Design review of the part built by this model. Coordinates are the model's own, in mm. A direction names the side the tool comes from. Give positions to 0.01 mm unless a question says otherwise; leave off trailing zeros. Loops run counter-clockwise (first coordinate to the right, second up) from the corner with the lowest first, then second, coordinate; pieces in that order, holes last. Notation, with made-up numbers: (74, 68.5) - (80, 68.5) arc R22 cw to (80, 88.5) - close; hole circle Ø1 at (9.25, 70). An arc over 180 degrees is marked (long way). Write each question's results on one line, items separated by ' | '.
from build123d import *

# Parameters (mm, degrees)
F0_W      = 7.9375
F0_H      = 31.75
F0_R      = 2.38125
F1_DEPTH  = 9.525
F2_DEPTH  = 11.1125
F3_W      = 3.175
F3_H      = 2.38125
F4_DEPTH  = 3.175
F5_W      = 1.5875
F5_H      = 6.35
F6_DEPTH  = 6.35
F7_DEPTH  = 1.5875
F8_R      = 1.5875
F9_DEPTH  = 0.79375
F10_R     = 1.5875
F11_DEPTH = 0.79375


with BuildPart() as f1:
    # F0 (on Top) → F1 (new body)
    with BuildSketch(Plane.XY):
        Rectangle(F0_W, F0_H)
        with Locations((0, -11.90625)):
            Circle(F0_R, mode=Mode.SUBTRACT)
        with Locations((0, -3.96875)):
            Circle(F0_R, mode=Mode.SUBTRACT)
        with Locations((0, 3.96875)):
            Circle(F0_R, mode=Mode.SUBTRACT)
        with Locations((0, 11.90625)):
            Circle(F0_R, mode=Mode.SUBTRACT)
    extrude(amount=F1_DEPTH)

    # F0 (on Top) → F2 (join)
    with BuildSketch(Plane.XY):
        with Locations((0, 11.90625)):
            Circle(F0_R)
        with Locations((0, -11.90625)):
            Circle(F0_R)
        with Locations((0, 3.96875)):
            Circle(F0_R)
        with Locations((0, -3.96875)):
            Circle(F0_R)
    extrude(amount=F2_DEPTH)

    # F3 (on Right) → F4 (join, symmetric)
    with BuildSketch(Plane.YZ):
        with Locations((-17.4625, 6.746875)):
            Rectangle(F3_W, F3_H)
        with Locations((-17.4625, 4.365625)):
            Rectangle(F3_W, F3_H)
        with BuildLine():
            Line((-21.43125, 5.55625), (-19.05, 5.55625))
            Line((-19.05, 5.55625), (-19.05, 7.9375))
            ThreePointArc((-19.05, 7.9375), (-20.733798, 7.240048), (-21.43125, 5.55625))
        make_face()
        with BuildLine():
            Line((-19.05, 3.175), (-19.05, 5.55625))
            Line((-19.05, 5.55625), (-21.43125, 5.55625))
            ThreePointArc((-21.43125, 5.55625), (-20.733798, 3.872452), (-19.05, 3.175))
        make_face()
    extrude(amount=F4_DEPTH, both=True)

    # F5 (on face) → F6 (cut)
    with BuildSketch(Plane.XY.offset(7.9375)):
        with Locations((0.79375, -19.05)):
            Rectangle(F5_W, F5_H)
        with Locations((-0.79375, -19.05)):
            Rectangle(F5_W, F5_H)
    extrude(amount=-F6_DEPTH, mode=Mode.SUBTRACT)

    # F3 (on Right) → F7 (join, symmetric)
    with BuildSketch(Plane.YZ):
        Polygon((15.875, 8.73125), (15.875, 5.55625), (22.225, 5.55625), (22.225, 7.9375), align=None)
        Polygon((22.225, 5.55625), (15.875, 5.55625), (15.875, 2.38125), (22.225, 3.175), align=None)
    extrude(amount=F7_DEPTH, both=True)

    # F8 (on face) → F9 (cut)
    with BuildSketch(Plane.YZ.offset(1.5875)):
        with Locations((19.05, 5.55625)):
            Circle(F8_R)
    extrude(amount=-F9_DEPTH, mode=Mode.SUBTRACT)

    # F10 (on face) → F11 (cut)
    with BuildSketch(Plane(origin=(-1.5875, 0, 0), x_dir=(0, -1, 0), z_dir=(-1, 0, 0))):
        with Locations((-19.05, 5.55625)):
            Circle(F10_R)
    extrude(amount=-F11_DEPTH, mode=Mode.SUBTRACT)


solid = f1.part
(1) Insertion check: P1, Ø4, axis at y = -19, z = 6, coming from the +X side (3 decimals); P2, Ø4, axis at y = 19.05, z = 5.56, coming from the +X side; P3, Ø0.8, axis at x = -2.5, y = -18, coming from the +Z side. Each pin has a flat end and moves straight along its axis. Give the tip position at first contact, or say it passes through.
Answers below:
P1: x = 3.175 | P2: x = 1.59 | P3: z = 7.94
(2) Wall thickness on line 1 along Y through (x, z) = (1.25, 10.5); line 2 along Y through (x, z) = (-1.75, 9) (3 decimals); line 3 along Z through (x, y) = (2.75, -19) (1 decimal): over which ranges is each line inside the solid? List them lowest first. Write a range as from..to.
Answers below:
line 1: -13.93..-9.88, -6..-1.94, 1.94..6, 9.88..13.93 | line 2: -15.875..15.875 | line 3: 3.2..7.9
(3) Take a section at C-C on z = 6.75. Give the boundary of the cut face in (x, y) (1 decimal), plus the area to 3 significant figures.
Answers below:
outline: (-4, -15.9) - (-3.2, -15.9) - (-3.2, -21.1) - (-1.6, -21.1) - (-1.6, -15.9) - (1.6, -15.9) - (1.6, -21.1) - (3.2, -21.1) - (3.2, -15.9) - (4, -15.9) - (4, 15.9) - (1.6, 15.9) - (1.6, 18) - (0.8, 18) - (0.8, 20.1) - (1.6, 20.1) - (1.6, 22.2) - (-1.6, 22.2) - (-1.6, 20.1) - (-0.8, 20.1) - (-0.8, 18) - (-1.6, 18) - (-1.6, 15.9) - (-4, 15.9) - close | area: 285 mm2
(4) Take a section at D-D on y = 2. Give the boundary of the cut face in (x, z) (1 decimal), plus the area to 3 significant figures.
Answers below:
outline: (-4, 0) - (4, 0) - (4, 9.5) - (1.3, 9.5) - (1.3, 11.1) - (-1.3, 11.1) - (-1.3, 9.5) - (-4, 9.5) - close | area: 79.9 mm2
(5) Draft analysis for pull direction Y (two halves, no side actions). For faces 1 (the cylindrical face through (1.196, 17.464, 5.626)), 2 (the flat face through (0, 22.225, 6)), 3 (the flat face through (1.588, 18, 7)), state which applies: pulls with the +Y half, pulls with the -Y half, needs draft (parallel to the pull), parting line crosses it, or undercut.
Answers below:
face 1: undercut | face 2: pulls with the +Y half | face 3: needs draft
(6) Take a section at B-B on y = 19.05. Give the boundary of the cut face in (x, z), plus the area to 3 significant figures.
Answers below:
outline: (-1.59, 2.78) - (1.59, 2.78) - (1.59, 3.97) - (0.79, 3.97) - (0.79, 7.14) - (1.59, 7.14) - (1.59, 8.33) - (-1.59, 8.33) - (-1.59, 7.14) - (-0.79, 7.14) - (-0.79, 3.97) - (-1.59, 3.97) - close | area: 12.6 mm2
(7) Tool access review of faces 4 (the flat face through (0.794, 19, 6)), 5 (the flat face through (-2, -17, 7.938)), 6 (the flat face through (0, 0, 9.525)): name each direction out of +Z, -Z, +X, -X, +Y, -Y from which nothing blocks a thin tool from reaching the whole face with its end or side.
Answers below:
face 4: +X | face 5: +Z, +X, -X, -Y | face 6: +Z
